Could you check a few things on this drawing? It's one solid part, dimensions in mm from its lowest x, y, z. Give positions to 0.01 mm unless a question says otherwise; leave off trailing zeros. Loops run counter-clockwise (first coordinate to the right, second up) from the corner with the lowest first, then second, coordinate; pieces in that order, holes last. Notation, with made-up numbers: M 74.5,14 L 82.5,14 A25 cw 82.5,29 Z; hole C 1.25,64.25 d4. An arc over 180 degrees is marked long. Answer in a Markdown table with one row per item. Add a question column.
1. I need wall thicknesses on line 1 along X through (y, z) = (12.25, 25); line 2 along Y through (x, z) = (19.5, 39); line 3 along Y through (x, z) = (3.25, 9). Which ranges of each line are inside material? Lowest first, please. Write a range as from..to.
2. If we section it at B-B on x = 6.75: List the corners of the cut face in (y, z) for me.
3. I'm going to push flat-ended pins straight in: pin 1 Ø1.5 at (x, z) = (20, 37.5) entering from -Y; pin 2 Ø6 at (y, z) = (6.5, 41) entering from +X; pin 3 Ø4 at (y, z) = (18, 23) entering from +X. Where does each tip first touch, or does it pass through?
4. If we section it at C-C on y = 7: List the corners of the cut face in (x, z) for me, then the cut area to 3 significant figures.
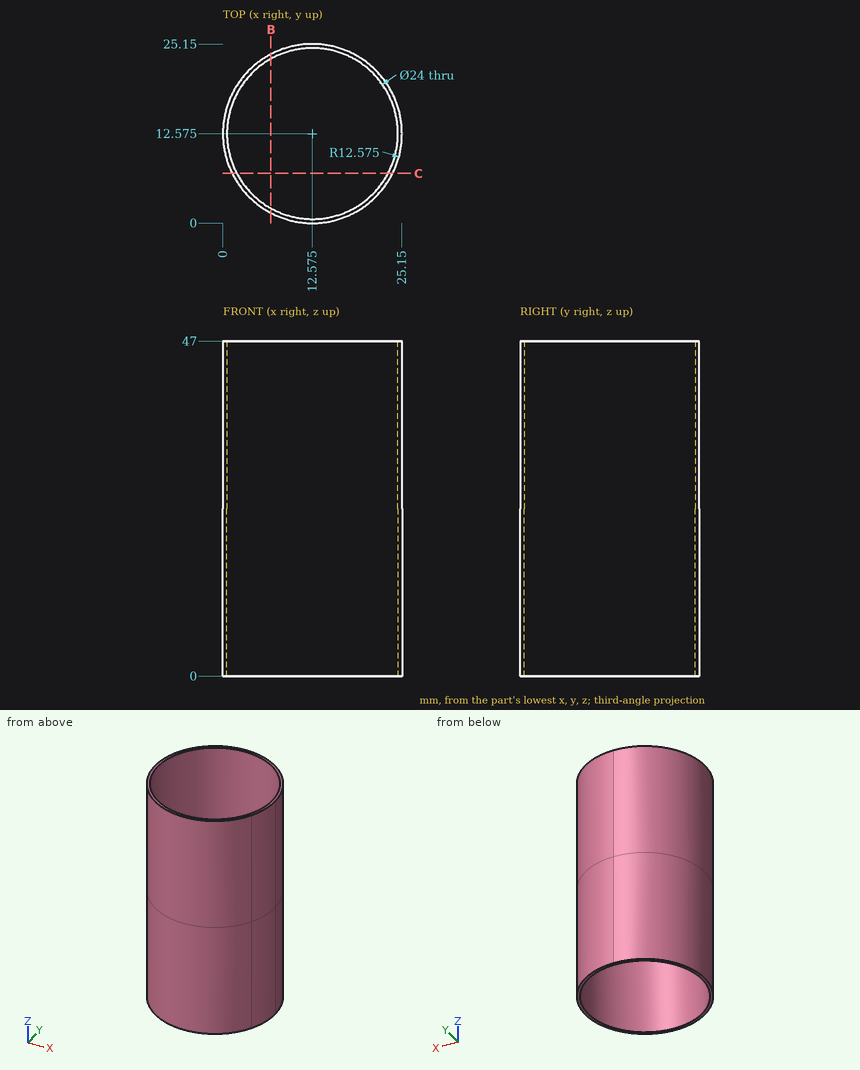
Results:
| question | item | result |
|---|---|---|
| 1 | line 1 | 0..0.58, 24.57..25.15 |
| 1 | line 2 | 2.08..2.77, 22.38..23.07 |
| 1 | line 3 | 4.14..5.02, 20.13..21.01 |
| 2 | outline | M 1.43,0 L 2.08,0 L 2.08,47 L 1.43,47 Z; M 23.07,0 L 23.72,0 L 23.72,47 L 23.07,47 Z |
| 3 | pin 1 | y = 1.92 |
| 3 | pin 2 | x = 24.77 |
| 3 | pin 3 | x = 24.67 |
| 4 | outline | M 1.3,0 L 1.95,0 L 1.95,47 L 1.3,47 Z; M 23.2,0 L 23.85,0 L 23.85,47 L 23.2,47 Z |
| 4 | area | 60.7 mm2 |
